Solid Edge part; units mm, degrees
sketch "Sketch1" plane through (0, 0, 0) normal (0, 0, 1) x (1, 0, 0)
  circle A0 centre (0, 0) radius 9.135
extrude "Protrusion1" add sketch "Sketch1" along normal blind 9
sketch "Sketch2" plane through (0, 0, 9) normal (0, 0, 1) x (1, 0, 0)
  line L0 (0, -3.4641) -> (-3, -1.7321)
  line L1 (-3, -1.7321) -> (-3, 1.7321)
  line L2 (-3, 1.7321) -> (0, 3.4641)
  line L3 (0, 3.4641) -> (3, 1.7321)
  line L4 (3, 1.7321) -> (3, -1.7321)
  line L5 (3, -1.7321) -> (0, -3.4641)
extrude "Cutout1" cut sketch "Sketch2" against normal blind 4.5
sketch "Sketch3" plane through (0, 0, 0) normal (0, 0, -1) x (0, 1, 0)
  circle A0 centre (0, 0) radius 6
extrude "Protrusion2" add sketch "Sketch3" along normal blind 30
sketch "Sketch4" plane through (0, 0, -30) normal (0, 0, -1) x (0, 1, 0)
  circle A0 centre (0, 0) radius 5
extrude "Protrusion3" add sketch "Sketch4" along normal blind 16
chamfer "Chamfer1" distance 0.5 angle 45 1 edges at (0, -5, -46)
properties part number "108080"
Geometry: final body of the model. Coordinates: model frame, mm. A direction names the side the tool comes from. Give positions to 0.01 mm unless a question says otherwise; leave off trailing zeros. Loops run counter-clockwise (first coordinate to the right, second up) from the corner with the lowest first, then second, coordinate; pieces in that order, holes last. Notation, with made-up numbers: (-19, 17.5) -> (36, 17.5) arc R23 ccw to (36, 50.5) -> close; hole circle Ø11 at (13, 6). An arc over 180 degrees is marked (long way). Return JSON: item names as keys, results as strings.
Item 1: Section D-D, the plane z = 3. Output: boundary loops of the cut face in (x, y) (3 decimals).
Filled in:
{"outline": "circle Ø18.27 at (0, 0)"}
Item 2: Pin query (flat end, axial travel): P1, Ø6, axis at x = -2.5, z = -31, coming from the -Y side; P2, Ø4, axis at x = 5.5, y = 7, coming from the -Z side; P3, Ø1.5, axis at y = 4, z = -22.5, coming from the +X side. Return the tip coordinate at first contact, or that it passes through.
Filled in:
{"P1": "y = -6", "P2": "z = 0", "P3": "x = 5.04"}
Item 3: Mould query, pull axis Y, two halves, no side actions, for faces 4 (the flat face through (2, -6, 0)), 5 (the flat face through (-3, 0, 7)), 6 (the cylindrical face through (4.88, -1.08, -37.64)). Classes: released by +Y, released by -Y, zero draft, split by the parting line, or undercut.
Filled in:
{"face 4": "zero draft", "face 5": "undercut", "face 6": "split by the parting line"}
Item 4: Section B-B, the plane z = -25. Output: boundary loops of the cut face in (x, y), plus the area to 3 significant figures.
Filled in:
{"outline": "circle Ø12 at (0, 0)", "area": "113 mm^2"}
Item 5: Access query for faces 1 (the flat face through (4, 4, -30)), 2 (the flat face through (0, 0, -46)), 3 (the flat face through (-1.5, 2.6, 6.8)). Directions: +Z, -Z, +X, -X, +Y, -Y. A direction counts if a zero-diameter tool reaches every point of the face in a straight line with its end or side. Return the directions, or none.
Filled in:
{"face 1": "-Z", "face 2": "-Z, +X, -X, +Y, -Y", "face 3": "+Z"}
Item 6: Line query: line 1 (Z direction, x = -3.5, y = 4.25); line 2 (Z direction, x = -0.5, y = 0.25); line 3 (X direction, y = 0, z = -25). Output: solid intervals per line, ascending.
Filled in:
{"line 1": "-30 to 9", "line 2": "-46 to 4.5", "line 3": "-6 to 6"}
Item 7: Section C-C, the plane x = -8. Output: boundary loops of the cut face in (y, z).
Filled in:
{"outline": "(-4.41, 0) -> (4.41, 0) -> (4.41, 9) -> (-4.41, 9) -> close"}
Item 8: Section A-A, the plane y = 0. Output: boundary loops of the cut face in (x, z) (3 decimals).
Filled in:
{"outline": "(-9.135, 0) -> (-6, 0) -> (-6, -30) -> (-5, -30) -> (-5, -45.5) -> (-4.5, -46) -> (4.5, -46) -> (5, -45.5) -> (5, -30) -> (6, -30) -> (6, 0) -> (9.135, 0) -> (9.135, 9) -> (3, 9) -> (3, 4.5) -> (-3, 4.5) -> (-3, 9) -> (-9.135, 9) -> close"}
